Model file for the job. Use its own axes, mm. Face numbers are marked on the shaded views. A direction names the side the tool comes from. Round coordinates to 2 decimals unless told otherwise and drop trailing zeros. Order: outer loops, then holes, each group sorted by start corner. A loop starts at its lowest first (then second) coordinate and runs counter-clockwise, first axis right, second up. Notation, with made-up numbers: (24.25, 89.25) - (80.25, 89.25) arc R25 ccw to (80.25, 110.25) - close; hole circle Ø2 at (45.5, 18.5). An arc over 180 degrees is marked (long way). Use one line per item in the form item = value.
from build123d import *

# Parameters (mm, degrees)
BOSS_EXTRUDE1_DEPTH = 5
BOSS_EXTRUDE2_DEPTH = 2
SKETCH4_W           = 24
SKETCH4_H           = 3
BOSS_EXTRUDE3_DEPTH = 49
CUT_EXTRUDE1_REACH  = 10.25
SKETCH5_R           = 1.75
SKETCH5_W           = 8
SKETCH5_H           = 14
SKETCH6_R           = 3.25
SKETCH6_R_2         = 1.75
BOSS_EXTRUDE4_DEPTH = 3


with BuildPart() as part:
    # Sketch1 → Boss-Extrude1 (new body)
    with BuildSketch(Plane(origin=(0, 0, 0), x_dir=(1, 0, 0), z_dir=(0, 1, 0))):
        with BuildLine():
            Line((-18.25, 6.75), (18.25, 6.75))
            ThreePointArc((18.25, 6.75), (20.371320344, 5.871320344), (21.25, 3.75))
            Line((21.25, 3.75), (21.25, -3.75))
            ThreePointArc((21.25, -3.75), (20.371320344, -5.871320344), (18.25, -6.75))
            Line((18.25, -6.75), (-18.25, -6.75))
            ThreePointArc((-18.25, -6.75), (-20.371320344, -5.871320344), (-21.25, -3.75))
            Line((-21.25, -3.75), (-21.25, 3.75))
            ThreePointArc((-21.25, 3.75), (-20.371320344, 5.871320344), (-18.25, 6.75))
        make_face()
        with BuildLine():
            Line((16.260111444, 2.189943648), (0.716289014, 3.681276533))
            ThreePointArc((0.716289014, 3.681276533), (0, 3.715559552), (-0.716289014, 3.681276533))
            Line((-0.716289014, 3.681276533), (-16.260111444, 2.189943648))
            ThreePointArc((-16.260111444, 2.189943648), (-18.25, 0), (-16.260111444, -2.189943648))
            Line((-16.260111444, -2.189943648), (-0.716289014, -3.681276533))
            ThreePointArc((-0.716289014, -3.681276533), (0, -3.715559552), (0.716289014, -3.681276533))
            Line((0.716289014, -3.681276533), (16.260111444, -2.189943648))
            ThreePointArc((16.260111444, -2.189943648), (18.25, 0), (16.260111444, 2.189943648))
        make_face(mode=Mode.SUBTRACT)
    extrude(amount=BOSS_EXTRUDE1_DEPTH)

    # Sketch2 → Boss-Extrude2 (add)
    with BuildSketch(Plane.XZ):
        with BuildLine():
            Line((-16.260111444, 2.189943648), (-6, 3.174337395))
            Line((-6, 3.174337395), (-6, -3.174337395))
            Line((-6, -3.174337395), (-16.260111444, -2.189943648))
            ThreePointArc((-16.260111444, -2.189943648), (-18.25, 0), (-16.260111444, 2.189943648))
        make_face()
        with BuildLine():
            Line((6, -3.174337395), (16.260111444, -2.189943648))
            ThreePointArc((16.260111444, -2.189943648), (18.25, 0), (16.260111444, 2.189943648))
            Line((16.260111444, 2.189943648), (6, 3.174337395))
            Line((6, 3.174337395), (6, -3.174337395))
        make_face()
    extrude(amount=-BOSS_EXTRUDE2_DEPTH)

    # Sketch4 → Boss-Extrude3 (add)
    with BuildSketch(Plane.XZ):
        Rectangle(SKETCH4_W, SKETCH4_H)
    extrude(amount=BOSS_EXTRUDE3_DEPTH)

    # Sketch5 → Cut-Extrude1 (cut, up to next)
    with BuildSketch(Plane(origin=(0, 0, -1.5), x_dir=(-1, 0, 0), z_dir=(0, 0, -1)), mode=Mode.PRIVATE) as cut_extrude1_sk1:
        with Locations((7.85, -44.85)):
            Circle(SKETCH5_R)
    cut_extrude1_tool1 = extrude(cut_extrude1_sk1.sketch, amount=-CUT_EXTRUDE1_REACH, mode=Mode.PRIVATE) & part.part
    add(cut_extrude1_tool1.solids().sort_by_distance((-7.85, -44.85, -1.5))[0], mode=Mode.SUBTRACT)
    # Sketch5 → Cut-Extrude1 (cut, up to next)
    with BuildSketch(Plane(origin=(0, 0, -1.5), x_dir=(-1, 0, 0), z_dir=(0, 0, -1)), mode=Mode.PRIVATE) as cut_extrude1_sk2:
        with Locations((-7.85, -44.85)):
            Circle(SKETCH5_R)
    cut_extrude1_tool2 = extrude(cut_extrude1_sk2.sketch, amount=-CUT_EXTRUDE1_REACH, mode=Mode.PRIVATE) & part.part
    add(cut_extrude1_tool2.solids().sort_by_distance((7.85, -44.85, -1.5))[0], mode=Mode.SUBTRACT)
    # Sketch5 → Cut-Extrude1 (cut, up to next)
    with BuildSketch(Plane(origin=(0, 0, -1.5), x_dir=(-1, 0, 0), z_dir=(0, 0, -1)), mode=Mode.PRIVATE) as cut_extrude1_sk3:
        with Locations((-7.85, -4.15)):
            Circle(SKETCH5_R)
    cut_extrude1_tool3 = extrude(cut_extrude1_sk3.sketch, amount=-CUT_EXTRUDE1_REACH, mode=Mode.PRIVATE) & part.part
    add(cut_extrude1_tool3.solids().sort_by_distance((7.85, -4.15, -1.5))[0], mode=Mode.SUBTRACT)
    # Sketch5 → Cut-Extrude1 (cut, up to next)
    with BuildSketch(Plane(origin=(0, 0, -1.5), x_dir=(-1, 0, 0), z_dir=(0, 0, -1)), mode=Mode.PRIVATE) as cut_extrude1_sk4:
        with Locations((7.85, -4.15)):
            Circle(SKETCH5_R)
    cut_extrude1_tool4 = extrude(cut_extrude1_sk4.sketch, amount=-CUT_EXTRUDE1_REACH, mode=Mode.PRIVATE) & part.part
    add(cut_extrude1_tool4.solids().sort_by_distance((-7.85, -4.15, -1.5))[0], mode=Mode.SUBTRACT)
    # Sketch5 → Cut-Extrude1 (cut, up to next)
    with BuildSketch(Plane(origin=(0, 0, -1.5), x_dir=(-1, 0, 0), z_dir=(0, 0, -1)), mode=Mode.PRIVATE) as cut_extrude1_sk5:
        with Locations((8, -24.5)):
            Rectangle(SKETCH5_W, SKETCH5_H)
    cut_extrude1_tool5 = extrude(cut_extrude1_sk5.sketch, amount=-CUT_EXTRUDE1_REACH, mode=Mode.PRIVATE) & part.part
    add(cut_extrude1_tool5.solids().sort_by_distance((-8, -24.5, -1.5))[0], mode=Mode.SUBTRACT)

    # Sketch6 → Boss-Extrude4 (add)
    with BuildSketch(Plane(origin=(0, 0, -1.5), x_dir=(-1, 0, 0), z_dir=(0, 0, -1))):
        with Locations((-7.85, -4.15)):
            Circle(SKETCH6_R)
        with Locations((-7.85, -4.15)):
            Circle(SKETCH6_R_2, mode=Mode.SUBTRACT)
        with Locations((7.85, -4.15)):
            Circle(SKETCH6_R)
        with Locations((7.85, -4.15)):
            Circle(SKETCH6_R_2, mode=Mode.SUBTRACT)
        with Locations((7.85, -44.85)):
            Circle(SKETCH6_R)
        with Locations((7.85, -44.85)):
            Circle(SKETCH6_R_2, mode=Mode.SUBTRACT)
        with Locations((-7.85, -44.85)):
            Circle(SKETCH6_R)
        with Locations((-7.85, -44.85)):
            Circle(SKETCH6_R_2, mode=Mode.SUBTRACT)
    extrude(amount=BOSS_EXTRUDE4_DEPTH)


solid = part.part
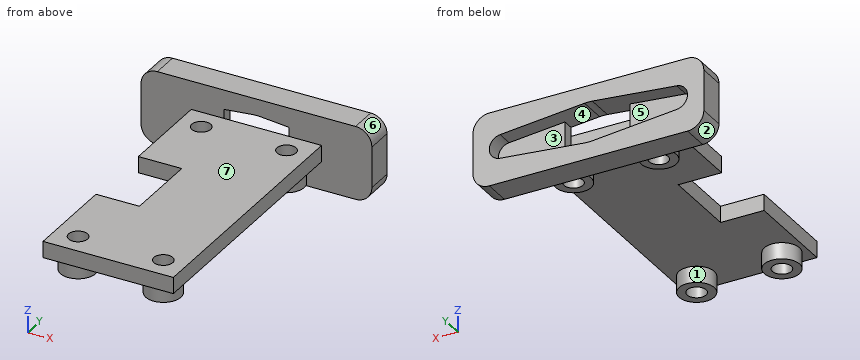
(1) Pin check, flat tips, straight feed: pin 1 (2 mm diameter, centred on x = 2, y = -10, fed in from -Z); pin 2 (3 mm diameter, centred on x = -8.5, y = -3.5, fed in from -Z); pin 3 (6 mm diameter, centred on y = -5, z = -4, fed in from +X). Stop position of each tip, or through.
Report:
pin_1 = -1.5
pin_2 = -4.5
pin_3 = 12
(2) Pull direction X, two halves, no side cores. Call the marked faces 4, 5, 6 and 7: released by +X, released by -X, zero draft, split by the parting line, or undercut.
Report:
face_4 = undercut
face_5 = undercut
face_6 = released by +X
face_7 = zero draft
(3) Probe probe 1 along Y at (x, z) = (-7.85, -2.85); probe 2 along Y at (x, z) = (-7.85, -3.65); probe 3 along Y at (x, z) = (7.85, 0.45). List the from-to ranges inside material, lowest first. Write a range as [from, to].
Report:
probe_1 = [-48.1, -46.6], [-43.1, -41.6], [-7.4, -5.9], [-2.4, -0.9], [0, 2]
probe_2 = [-48.1, -46.6], [-43.1, -41.6], [-7.4, -5.9], [-2.4, -0.9], [0, 5]
probe_3 = [-49, -46.6], [-43.1, -5.9], [-2.4, 2]
(4) Slice it at A-A on y = -44.85. Give the cut face in (x, z), then the cut area to 3 significant figures.
Report:
outline = (-12, -1.5) - (-11.1, -1.5) - (-11.1, -4.5) - (-9.6, -4.5) - (-9.6, 1.5) - (-12, 1.5) - close; (-6.1, -4.5) - (-4.6, -4.5) - (-4.6, -1.5) - (4.6, -1.5) - (4.6, -4.5) - (6.1, -4.5) - (6.1, 1.5) - (-6.1, 1.5) - close; (9.6, -4.5) - (11.1, -4.5) - (11.1, -1.5) - (12, -1.5) - (12, 1.5) - (9.6, 1.5) - close
area = 69.0 mm2
(5) Slice it at D-D on y = -10.5. Give the cut face in (x, z), then the cut area to 3 significant figures.
Report:
outline = (-12, -1.5) - (12, -1.5) - (12, 1.5) - (-12, 1.5) - close
area = 72.0 mm2
(6) Slice it at C-C on x = -7.85. Count the separate pieces of the cut face and the enclosed holes in it, then the cut area to 3 significant figures.
Report:
separate_pieces = 4
enclosed_holes = 0
area = 152 mm2
(7) Slice it at B-B on x = 4. Give the cut face in (y, z).
Report:
outline = (-49, -1.5) - (0, -1.5) - (0, 1.5) - (-49, 1.5) - close; (0, -6.75) - (5, -6.75) - (5, -3.37) - (0, -3.37) - close; (0, 3.37) - (5, 3.37) - (5, 6.75) - (0, 6.75) - close
(8) Tool access for the marked faces 1, 2 and 3: list every direction of +Z, -Z, +X, -X, +Y, -Y with a clear straight run to the whole face (end or side of a thin tool).
Report:
face_1 = -Z
face_2 = -Z, -X, +Y, -Y
face_3 = +Y
